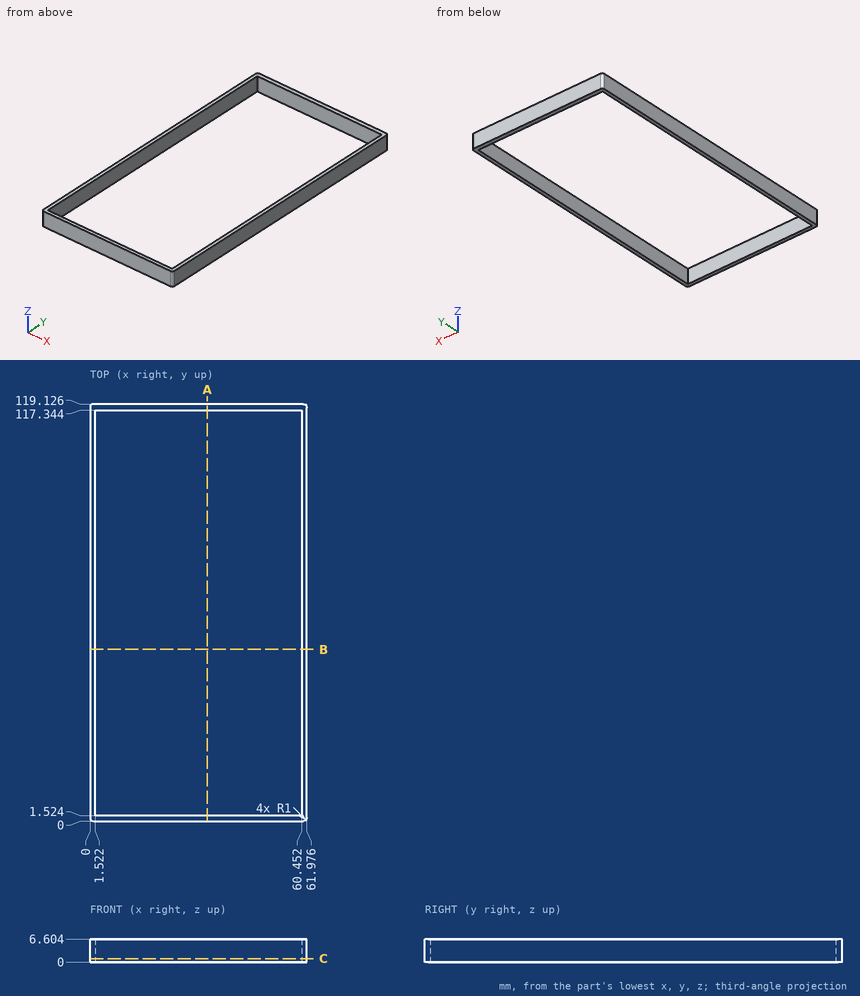
Study the drawing (mm; zero at the part's minimum x, y, z) and answer. Give positions to 0.01 mm unless a question says otherwise; leave off trailing zeros. Write each loop counter-clockwise with the first axis right and the second up, starting at its lowest first coordinate (ties: lowest second). Pieces come first, ordered by that corner, then holes. Notation, with made-up numbers: (64, 64.25) -> (98, 64.25) arc R15 cw to (98, 84.25) -> close; hole circle Ø3 at (52.25, 39). An arc over 180 degrees is marked (long way). Answer in a Markdown table with one row per item.
1) Each of these flat-tipped pins is pushed along its axis until it touches: pin 1 Ø2 at (x, z) = (32.5, 2.5) entering from -Y; pin 2 Ø8 at (x, y) = (55, 52) entering from -Z. Where does it stop, or does it pass through?
Results list:
| item | result |
|---|---|
| pin 1 | y = 0 |
| pin 2 | through |
2) Section B-B on y = 49 is taken. Give the vertices of the cut face in (x, z).
Results list:
| item | result |
|---|---|
| outline | (0, 0) -> (1.52, 0) -> (1.52, 6.6) -> (0, 6.6) -> close; (60.45, 0) -> (61.98, 0) -> (61.98, 6.6) -> (60.45, 6.6) -> close |
3) Section A-A on x = 33.5 is taken. Give the vertices of the cut face in (y, z).
Results list:
| item | result |
|---|---|
| outline | (0, 0) -> (1.52, 0) -> (1.52, 6.6) -> (0, 6.6) -> close; (117.34, 0) -> (119.13, 0) -> (119.13, 6.6) -> (117.34, 6.6) -> close |
4) Straight lines are drawn through the part: line 1 (Y direction, x = 40, z = 2); line 2 (X direction, y = 97, z = 1). For each, find the intervals that lie inside material, in ascending order. Write a range as [from, to].
Results list:
| item | result |
|---|---|
| line 1 | [0, 1.52], [117.34, 119.13] |
| line 2 | [0, 1.52], [60.45, 61.98] |
5) Section C-C on z = 1 is taken. Give the vertices of the cut face in (x, y), plus the area to 3 significant figures.
Results list:
| item | result |
|---|---|
| outline | (0, 1) arc R1 ccw to (1, 0) -> (60.98, 0) arc R1 ccw to (61.98, 1) -> (61.98, 118.13) arc R1 ccw to (60.98, 119.13) -> (1, 119.13) arc R1 ccw to (0, 118.13) -> close; hole (1.52, 1.52) -> (60.45, 1.52) -> (60.45, 117.34) -> (1.52, 117.34) -> close |
| area | 557 mm^2 |
